Verification items for the finished model (mm, model axes). Round coordinates to 2 decimals unless told otherwise and drop trailing zeros. Write each loop counter-clockwise with the first axis right and the second up, starting at its lowest first coordinate (ties: lowest second). Pieces come first, ordered by that corner, then holes. Notation, with made-up numbers: (30, 34) -> (78, 34) arc R25 cw to (78, 72) -> close; hole circle Ø4 at (-9, 31.25). An arc over 180 degrees is marked (long way). Use CSV: the item, a comma, the result in double quotes.
```python
from build123d import *

# Parameters (mm, degrees)
SKETCH1_R           = 2.25
BOSS_EXTRUDE1_DEPTH = 10
M6_TAPPED_HOLE1_D   = 5


with BuildPart() as part:
    # Sketch1 → Boss-Extrude1 (new body)
    with BuildSketch(Plane(origin=(0, 0, 0), x_dir=(0, 1, 0), z_dir=(0, 0, 1))):
        with BuildLine():
            Line((68.412788105, 40), (-68.412788105, 40))
            ThreePointArc((-68.412788105, 40), (-75.483855917, 37.071067812), (-78.412788105, 30))
            Line((-78.412788105, 30), (-78.412788105, -30))
            ThreePointArc((-78.412788105, -30), (-75.483855917, -37.071067812), (-68.412788105, -40))
            Line((-68.412788105, -40), (68.412788105, -40))
            ThreePointArc((68.412788105, -40), (75.483855917, -37.071067812), (78.412788105, -30))
            Line((78.412788105, -30), (78.412788105, 30))
            ThreePointArc((78.412788105, 30), (75.483855917, 37.071067812), (68.412788105, 40))
        make_face()
        with Locations(Location((70, 20, 0), (0, 0, 270))):
            Circle(SKETCH1_R, mode=Mode.SUBTRACT)
        with Locations(Location((70, -20, 0), (0, 0, 90))):
            Circle(SKETCH1_R, mode=Mode.SUBTRACT)
        with Locations(Location((-70, -20, 0), (0, 0, 270))):
            Circle(SKETCH1_R, mode=Mode.SUBTRACT)
        with Locations(Location((-70, 20, 0), (0, 0, 90))):
            Circle(SKETCH1_R, mode=Mode.SUBTRACT)
    extrude(amount=BOSS_EXTRUDE1_DEPTH)

    # M6 Tapped Hole1 (through all)
    with Locations(Plane.XY.offset(10)):
        with Locations((-31.819805153, -31.819805153), (31.819805153, 31.819805153), (-31.819805153, 31.819805153), (31.819805153, -31.819805153)):
            Hole(M6_TAPPED_HOLE1_D / 2)


solid = part.part
```
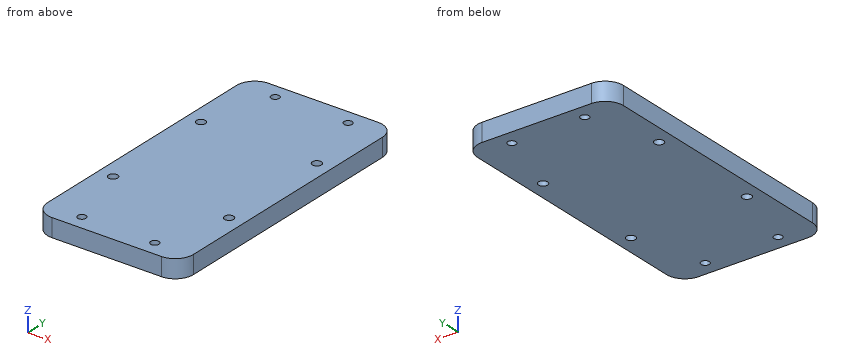
Q1. Go/stop test with a flat-tipped pin: P1, Ø12, axis at x = -31.5, y = 23, coming from the -Z side. Record where the tip stops, or that it passes through.
Filled in:
P1,"z = 0"
Q2. Section check B-B (y = -70). Record the cut outline in (x, z), plus the area to 3 significant figures.
Filled in:
outline,"(-39.87, 0) -> (-22.25, 0) -> (-22.25, 10) -> (-39.87, 10) -> close; (-17.75, 0) -> (17.75, 0) -> (17.75, 10) -> (-17.75, 10) -> close; (22.25, 0) -> (39.87, 0) -> (39.87, 10) -> (22.25, 10) -> close"
area,"707 mm²"
Q3. Section check C-C (z = 3). State how many separate pieces and enclosed holes the cut face has, plus the area to 3 significant figures.
Filled in:
separate pieces,"1"
enclosed holes,"8"
area,"12,300 mm²"
Q4. Material ranges on L1, parallel to Y at x = -20, z = 3; L2, parallel to X at y = -32, z = 1.25; L3, parallel to X at y = -71, z = 7.75, recorded low to high.
Filled in:
L1,"-78.41 to -72.25, -67.75 to 67.75, 72.25 to 78.41"
L2,"-40 to -34.31, -29.33 to 29.33, 34.31 to 40"
L3,"-39.66 to -22.02, -17.98 to 17.98, 22.02 to 39.66"
Q5. Section check A-A (x = 20). Record the cut outline in (y, z), plus the area to 3 significant figures.
Filled in:
outline,"(-78.41, 0) -> (-72.25, 0) -> (-72.25, 10) -> (-78.41, 10) -> close; (-67.75, 0) -> (67.75, 0) -> (67.75, 10) -> (-67.75, 10) -> close; (72.25, 0) -> (78.41, 0) -> (78.41, 10) -> (72.25, 10) -> close"
area,"1,480 mm²"
